Here's how the part is built. I have some questions about the finished solid (model axes, mm). Round coordinates to 2 decimals unless told otherwise and drop trailing zeros. Order: outer loops, then holes, each group sorted by start corner. A loop starts at its lowest first (then second) coordinate and runs counter-clockwise, first axis right, second up. Notation, with made-up numbers: (-40, 33) -> (9, 33) arc R27 ccw to (9, 59) -> close; hole circle Ø8 at (13.25, 83.5). An arc over 180 degrees is marked (long way). Use a Markdown table: item, result. Add a question column.
Autodesk Inventor part; units mm, degrees
ref_plane "Work Plane1" through (0, 4, 0) normal (0, 1, 0) x (1, 0, 0)
ref_plane "YZ Plane" through (0, 0, 0) normal (1, 0, 0) x (0, 1, 0)
ref_plane "XZ Plane" through (0, 0, 0) normal (0, 1, 0) x (-1, 0, 0)
sketch "Sketch2" plane through (0, 0, 0) normal (0, 1, 0) x (-1, 0, 0)
  line L0 (15, 29) -> (-15, 29)
  line L1 (-15, 29) -> (-15, -29)
  line L2 (-15, -29) -> (15, -29)
  line L3 (15, -29) -> (15, 29)
  line L4 (0, 0) -> (0, -29) construction
  line L5 (0, 0) -> (0, 29) construction
  line L6 (0, 0) -> (15, 0) construction
  line L7 (0, 0) -> (-15, 0) construction
  dimension "d45" = 30
  dimension "d46" = 58
extrude "Main Body Sketch" add sketch "Sketch2" along normal blind 4
ref_plane "Work Plane1" through (0, 4, 0) normal (0, 1, 0) x (1, 0, 0)
sketch "Sketch4" plane through (0, 4, 0) normal (0, 1, 0) x (1, 0, 0)
  circle A0 centre (0, -15) radius 7
  circle A1 centre (5, 17.5) radius 2.15
  circle A2 centre (-5, 17.5) radius 2.15
  line L0 (15, 29) -> (-15, 29)
  line L1 (-15, 29) -> (-15, -29)
  dimension "d85" = 30
  dimension "d87" = 4.3
  dimension "d88" = 4.3
  dimension "d90" = 10
  dimension "d96" = 14
  dimension "d97" = 44
  dimension "d98" = 15
  dimension "d100" = 11.5
  dimension "d101" = 11.5
extrude "Holes Cuts" cut sketch "Sketch4" against normal up to surface (4 mm away)
fillet "Fillet12" radius 4 2 edges at (-15, 2, -29) (15, 2, -29)
fillet "Fillet12" radius 15 2 edges at (15, 2, 29) (-15, 2, 29)
fillet "Fillet13" radius 1 12 edges at (10.6067, 4, 24.6067) (15, 4, -5.5) (13.8286, 4, -27.8286) (0, 4, -29) (-13.8286, 4, -27.8286) (-15, 4, -5.5) (15, 0, -5.5) (13.8286, 0, -27.8286) (0, 0, -29) (-13.8286, 0, -27.8286) (-15, 0, -5.5) (10.6067, 0, 24.6067)
equation "\"d46\" = AH"
equation "\"AH\" = 58"
equation "\"d57\" = TMROL"
equation "\"BD\" = 4"
properties part number "Side Attatchment"
(1) Please list where these lines run through material, in increasing order: probe 1 along X at (y, z) = (0.9, -17.5); probe 2 along Z at (x, y) = (0, 2.7); probe 3 along Z at (x, y) = (-3.25, 3.2). Write a range as from..to.
(2) I want a section at C-C on x = 5.75. State how many separate pieces and enclosed holes the cut face has, and give its area (3 significant figures).
(3) If we mould it in two halves opening along X, with no side actions, what happens to faces 1 (the cylindrical face through (-1.517, 2.028, 21.834)), 2 (the cylindrical face through (-14.699, 3.715, -5.227)), 3 (the cylindrical face through (13.859, 2.014, -27.797))? For each: pulls with the +X half, pulls with the -X half, needs draft (parallel to the pull), parting line crosses it, or undercut.
(4) I want a section at A-A on z = -17.5. List the corners of the cut face in (x, y) for me.
(5) I want a section at B-B on z = 11.5. List the corners of the cut face in (x, y) for me, and give its area (3 significant figures).
(6) I'm going to push flat-ended pins straight in: P1, Ø1, axis at x = -6, z = 0, coming from the -Y side; P2, Ø1.5, axis at x = 9, y = 3, coming from the +Z side. Where does each tip first touch, or does it pass through?
Output:
| question | item | result |
|---|---|---|
| 1 | probe 1 | -14.99..-7.15, -2.85..2.85, 7.15..14.99 |
| 1 | probe 2 | -29..8, 22..29 |
| 1 | probe 3 | -28.98..-18.75, -16.25..8.8, 21.2..28.62 |
| 2 | separate pieces | 3 |
| 2 | enclosed holes | 0 |
| 2 | area | 178 mm² |
| 3 | face 1 | undercut |
| 3 | face 2 | pulls with the -X half |
| 3 | face 3 | pulls with the +X half |
| 4 | outline | (-15, 1) arc R1 ccw to (-14, 0) -> (-7.15, 0) -> (-7.15, 4) -> (-14, 4) arc R1 ccw to (-15, 3) -> close; (-2.85, 0) -> (2.85, 0) -> (2.85, 4) -> (-2.85, 4) -> close; (7.15, 0) -> (14, 0) arc R1 ccw to (15, 1) -> (15, 3) arc R1 ccw to (14, 4) -> (7.15, 4) -> close |
| 5 | outline | (-15, 1) arc R1 ccw to (-14, 0) -> (-6.06, 0) -> (-6.06, 4) -> (-14, 4) arc R1 ccw to (-15, 3) -> close; (6.06, 0) -> (14, 0) arc R1 ccw to (15, 1) -> (15, 3) arc R1 ccw to (14, 4) -> (6.06, 4) -> close |
| 5 | area | 70.6 mm² |
| 6 | P1 | y = 0 |
| 6 | P2 | z = 26.53 |
